The listing builds one solid part. Answer for the finished solid, in the listing's coordinates (mm). A direction names the side the tool comes from. Coordinates: 2 decimals unless noted, no trailing zeros. Write each loop counter-clockwise with the first axis right and the second up, starting at its lowest first coordinate (ties: lowest second). Pieces come first, ordered by that corner, then holes.
(1) The part is cut by section C-C on x = -20. Determine the outline of the cut face in (y, z).
(2) The part is cut by section D-D on x = 30.5. Determine the outline of the cut face in (y, z), plus the area to 3 significant figures.
(3) The part is cut by section A-A on y = -0.9. Determine the outline of the cut face in (x, z).
(4) The part is cut by section B-B on z = -27. Determine the outline of the cut face in (x, y), plus the area to 3 significant figures.
(5) Straight lines are drawn through the part: line 1 (Y direction, x = 48.5, z = -15); line 2 (X direction, y = -0.7, z = 0.5); line 3 (X direction, y = -0.75, z = 6.5). For each, find the intervals that lie inside material, in ascending order.
(6) Which of the six approach directions +Z, -Z, +X, -X, +Y, -Y give full straight-line access (tool end or side, diameter ignored) to faces 1 (the flat face through (18.507, 1.127, -4.714)), 2 (the flat face through (47.239, -1.127, -3.945)), 3 (the flat face through (-35, 0, -6))?
from build123d import *

# Parameters (mm, degrees)
EXTRUDE1_DEPTH = 2.286
EXTRUDE2_DEPTH = 2.286


with BuildPart() as part:
    # Sketch1 → Extrude1 (new body)
    with BuildSketch(Plane(origin=(0, 0, 0), x_dir=(1, 0, 0), z_dir=(0, 1, 0))):
        with BuildLine():
            Line((-53.408275127, 37.75591133), (53.408275127, 37.75591133))
            ThreePointArc((53.408275127, 37.75591133), (57.169709098, 35.782910846), (57.684725289, 31.566766311))
            Line((57.684725289, 31.566766311), (36.497605157, -24.461395817))
            ThreePointArc((36.497605157, -24.461395817), (34.820154512, -26.605684768), (32.221154995, -27.416250797))
            Line((32.221154995, -27.416250797), (-32.221154995, -27.416250797))
            ThreePointArc((-32.221154995, -27.416250797), (-34.820154512, -26.605684768), (-36.497605157, -24.461395817))
            Line((-36.497605157, -24.461395817), (-57.684725289, 31.566766311))
            ThreePointArc((-57.684725289, 31.566766311), (-57.169709098, 35.782910846), (-53.408275127, 37.75591133))
        make_face()
    extrude(amount=-EXTRUDE1_DEPTH)

    # Sketch2 → Extrude2 (add)
    with BuildSketch(Plane(origin=(0, 0, 0), x_dir=(1, 0, 0), z_dir=(0, 1, 0))):
        Polygon((-12.739414216, -27.416250797), (12.739414216, -27.416250797), (24.438876252, 37.75591133), (-24.438876252, 37.75591133), align=None)
    extrude(amount=EXTRUDE2_DEPTH)


solid = part.part
Model answer:
1. outline: (-2.29, -37.76) - (2.29, -37.76) - (2.29, -13.03) - (0, -13.03) - (0, 27.42) - (-2.29, 27.42) - close
2. outline: (-2.29, -37.76) - (0, -37.76) - (0, 27.42) - (-2.29, 27.42) - close
2. area: 149 mm2
3. outline: (-57.68, -31.57) arc R4.57 ccw to (-53.41, -37.76) - (53.41, -37.76) arc R4.57 ccw to (57.68, -31.57) - (36.5, 24.46) arc R4.57 ccw to (32.22, 27.42) - (-32.22, 27.42) arc R4.57 ccw to (-36.5, 24.46) - close
4. outline: (-55.96, -2.29) - (55.96, -2.29) - (55.96, 0) - (22.51, 0) - (22.51, 2.29) - (-22.51, 2.29) - (-22.51, 0) - (-55.96, 0) - close
4. area: 359 mm2
5. line 1: y = -2.29 to 0
5. line 2: x = -45.56 to 45.56
5. line 3: x = -43.29 to 43.29
6. face 1: +Z, +X, +Y
6. face 2: +Z, +X, +Y, -Y
6. face 3: +Z, -X, +Y
